Check sheet for the modelled part. Datum: model origin and axes. Units: mm. Give positions to 0.01 mm unless a question says otherwise; leave off trailing zeros. Order: outer loops, then holes, each group sorted by start corner. A loop starts at its lowest first (then second) coordinate and runs counter-clockwise, first axis right, second up. Notation, with made-up numbers: (52, 89) -> (59, 89) arc R31 cw to (59, 119) -> close; hole circle Ø1 at (36.5, 42.25). An arc over 180 degrees is marked (long way). One line per question, with ' | ' between items.
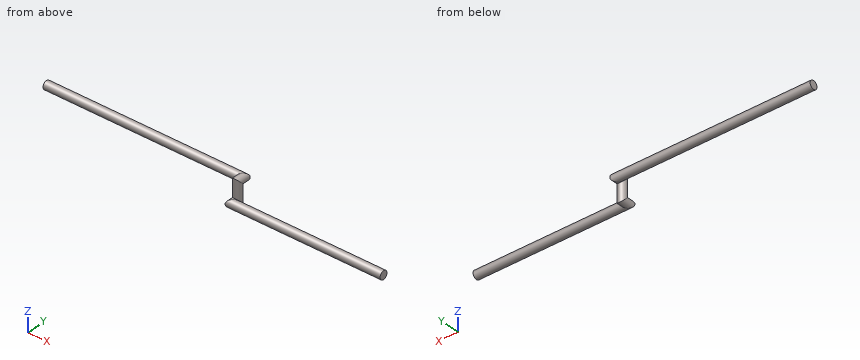
```python
from build123d import *

# Parameters (mm, degrees)
CROQUIS1_R = 13.7


with BuildPart() as part:
    # Barrer1: sweep along a curve in space
    with BuildLine() as barrer1_path:
        Line((0, 0, 0), (-500, 0, 0))
        Line((-500, 0, 0), (-500, 20, 0))
        Line((-500, 20, 0), (-500, 20, 60))
        Line((-500, 20, 60), (-500, 40, 60))
        Line((-500, 40, 60), (-1150, 40, 60))
    # Croquis1 → Barrer1 (sweep)
    with BuildSketch(Plane(origin=(0, 0, 0), x_dir=(0, 0, -1), z_dir=(1, 0, 0))):
        Circle(CROQUIS1_R)
    sweep(path=barrer1_path.line, transition=Transition.RIGHT)


solid = part.part
```
Q1. Section check C-C (z = 0). Enter the section's corners in (x, y).
Result sheet:
outline: (-513.7, -13.7) -> (0, -13.7) -> (0, 13.7) -> (-486.3, 13.7) -> (-486.3, 20) arc R13.7 ccw to (-513.7, 20) -> close
Q2. Thickness scan on line 1 (X direction, y = 39, z = 61.5); line 2 (X direction, y = 0, z = 2); line 3 (Y direction, x = -796.5, z = 62). Record the ranges inside material, lowest first.
Result sheet:
line 1: x = -1150 to -486.38 | line 2: x = -513.55 to 0 | line 3: y = 26.45 to 53.55
Q3. Section check A-A (x = -500). Enter the section's corners in (y, z).
Result sheet:
outline: (0, -13.7) -> (33.7, -13.7) -> (33.7, 46.3) -> (40, 46.3) arc R13.7 ccw to (40, 73.7) -> (6.3, 73.7) -> (6.3, 13.7) -> (0, 13.7) arc R13.7 ccw to start
Q4. Section check D-D (x = -781.5). Enter the section's corners in (y, z), and give its area (3 significant figures).
Result sheet:
outline: circle Ø27.4 at (40, 60) | area: 590 mm2
Q5. Depth check by flat-ended pin: pin 1 Ø6 at (y, z) = (20.5, 15.5) entering from +X; pin 2 Ø4 at (x, y) = (-782, 30) entering from -Z; pin 3 Ø5 at (y, z) = (12, -4.5) entering from -X. Enter the tip coordinate at first touch or a pass-through.
Result sheet:
pin 1: stops at x = -486.3 | pin 2: stops at z = 48.88 | pin 3: stops at x = -513.55
Q6. Section check B-B (z = 60). Enter the section's corners in (x, y), and give its area (3 significant figures).
Result sheet:
outline: (-1150, 26.3) -> (-513.7, 26.3) -> (-513.7, 20) arc R13.7 ccw to (-486.3, 20) -> (-486.3, 53.7) -> (-1150, 53.7) -> close | area: 18,700 mm2
